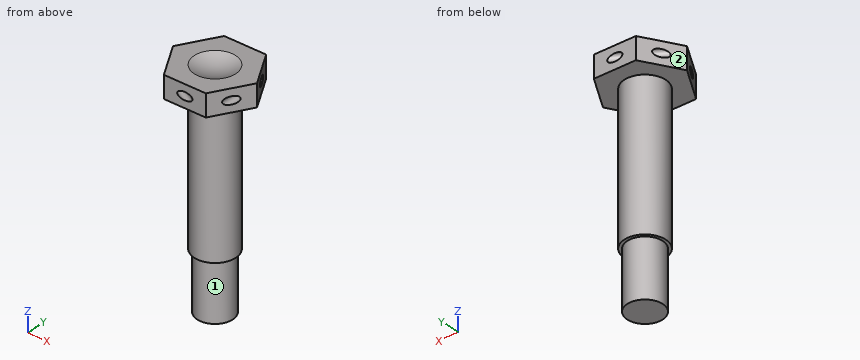
```python
from build123d import *

# Parameters (mm, degrees)
BOSS_EXTRUDE1_DEPTH = 3.3655
SKETCH2_R           = 3.1623
BOSS_EXTRUDE2_DEPTH = 22.225
SKETCH3_R           = 2.7051
BOSS_EXTRUDE3_DEPTH = 8.763
SKETCH5_R           = 0.5842
CUT_EXTRUDE1_DEPTH  = 33.129279639
CIRPATTERN1_COUNT   = 3


with BuildPart() as part:
    # Sketch1 → Boss-Extrude1 (new body)
    with BuildSketch(Plane.XY):
        Polygon((3.207902433, 5.55625), (-3.207902433, 5.55625), (-6.415804866, 0), (-3.207902433, -5.55625), (3.207902433, -5.55625), (6.415804866, 0), align=None)
    extrude(amount=BOSS_EXTRUDE1_DEPTH)

    # Sketch2 → Boss-Extrude2 (add)
    with BuildSketch(Plane(origin=(0, 0, 0), x_dir=(-1, 0, 0), z_dir=(0, 0, -1))):
        with Locations(Location((0, 0, 0), (0, 0, 180))):
            Circle(SKETCH2_R)
    extrude(amount=BOSS_EXTRUDE2_DEPTH)

    # Sketch3 → Boss-Extrude3 (add)
    with BuildSketch(Plane(origin=(0, 0, -22.225), x_dir=(-1, 0, 0), z_dir=(0, 0, -1))):
        Circle(SKETCH3_R)
    extrude(amount=BOSS_EXTRUDE3_DEPTH)

    # Sketch4 → Cut-Revolve1 (revolve, cut)
    with BuildSketch(Plane(origin=(0, 0, 0), x_dir=(0, 0, -1), z_dir=(1, 0, 0))):
        with BuildLine():
            Line((-3.3655, 0), (-3.3655, 3.1623))
            ThreePointArc((-3.3655, 3.1623), (-2.841803396, 1.619539554), (-2.664434968, 0))
            Line((-2.664434968, 0), (-3.3655, 0))
        make_face()
    revolve(axis=Axis((0, 0, 3.3655), (0, 0, -1)), mode=Mode.SUBTRACT)

    # Sketch5 → Cut-Extrude1 (cut, symmetric)
    with BuildSketch(Plane(origin=(0, 0, 0), x_dir=(1, 0, 0), z_dir=(0, 1, 0))):
        with Locations((4.81185365, -1.68275)):
            Circle(SKETCH5_R)
    cut_extrude1 = extrude(amount=CUT_EXTRUDE1_DEPTH, both=True, mode=Mode.SUBTRACT)

    # CirPattern1: Cut-Extrude1 ×3 about axis
    cirpattern1_axis = Axis((0, 0, -32.705675), (0, 0, 1))
    for i in range(1, CIRPATTERN1_COUNT):
        add(cut_extrude1.rotate(cirpattern1_axis, i * 360 / CIRPATTERN1_COUNT), mode=Mode.SUBTRACT)


solid = part.part
```
Geometry check sheet. Reference: the model listing, model coordinates, mm. Face numbers are marked on the shaded views. A direction names the side the tool comes from. Coordinates: 2 decimals unless noted, no trailing zeros. Order: outer loops, then holes, each group sorted by start corner. A loop starts at its lowest first (then second) coordinate and runs counter-clockwise, first axis right, second up.
Item 1: Scan lines: line 1 along Z through (x, y) = (3.5, 3); line 2 along Y through (x, z) = (0, -5); line 3 along Z through (x, y) = (-0.5, -4.75). Record each from-to range of solid material in increasing order.
Item 2: Depth check by flat-ended pin: pin 1 (3 mm diameter, centred on y = -4, z = -20, fed in from -X); pin 2 (3 mm diameter, centred on y = 0.5, z = -17, fed in from +X); pin 3 (1.3 mm diameter, centred on x = 4.81, z = 1.68, fed in from -Y); pin 4 (1 mm diameter, centred on x = 5, z = -11.5, fed in from +Y). Enter the tip coordinate at first touch or a pass-through.
Item 3: Section check C-C (z = -5). Enter the section's corners in (x, y), plus the area to 3 significant figures.
Item 4: Tool access check on the marked faces 1 and 2. Record the directions out of +Z, -Z, +X, -X, +Y, -Y that give a thin tool (end or side, any length) a straight path to the whole face; none if there is none.
Item 5: Section check A-A (y = -0.75). Enter the section's corners in (x, z) (1 decimal), plus the area to 3 significant figures.
Item 6: Section check B-B (z = -23). Enter the section's corners in (x, y).
Check sheet entries:
1. line 1: z = 0 to 3.37
1. line 2: y = -3.16 to 3.16
1. line 3: z = 0 to 1.31, 2.06 to 3.37
2. pin 1: stops at x = -1.94
2. pin 2: stops at x = 3.16
2. pin 3: stops at y = -3.91
2. pin 4: passes through
3. outline: circle Ø6.32 at (0, 0)
3. area: 31.4 mm2
4. face 1: -Z
4. face 2: +Z, -Z, -X, +Y
5. outline: (-6, 0) - (-3.1, 0) - (-3.1, -22.2) - (-2.6, -22.2) - (-2.6, -31) - (2.6, -31) - (2.6, -22.2) - (3.1, -22.2) - (3.1, 0) - (6, 0) - (6, 3.4) - (3.1, 3.4) arc R7.4 cw to (-3.1, 3.4) - (-6, 3.4) - close; hole circle Ø1.2 at (4.8, 1.7)
5. area: 219 mm2
6. outline: circle Ø5.41 at (0, 0)
